Autodesk Inventor part; units mm, degrees
ref_plane "YZ Plane" through (0, 0, 0) normal (1, 0, 0) x (0, 1, 0)
ref_plane "XZ Plane" through (0, 0, 0) normal (0, 1, 0) x (-1, 0, 0)
ref_plane "XY Plane" through (0, 0, 0) normal (0, 0, 1) x (1, 0, 0)
sketch "Boceto1" plane through (0, 0, 0) normal (0, 0, 1) x (1, 0, 0)
  point P0 (0, 0)
sketch "Boceto2" plane through (0, 0, 0) normal (0, 0, 1) x (1, 0, 0)
  line L0 (-7.0268, -6.2798) -> (7.0268, -6.2798)
  line L1 (7.0268, -6.2798) -> (7.0268, 6.2798)
  line L2 (7.0268, 6.2798) -> (-7.0268, 6.2798)
  line L3 (-7.0268, 6.2798) -> (-7.0268, -6.2798)
  line L4 (-7.0268, -6.2798) -> (7.0268, 6.2798) construction
  line L5 (7.0268, -6.2798) -> (-7.0268, 6.2798) construction
  line L6 (-9.5542, -8.5385) -> (-9.5542, 8.5385)
  line L7 (-9.5542, 8.5385) -> (38.1222, 8.5385)
  line L8 (38.1222, 8.5385) -> (38.1222, -8.5385)
  line L9 (38.1222, -8.5385) -> (-9.5542, -8.5385)
  point P0 (0, 0)
extrude "Extrusión1" add sketch "Boceto2" along normal blind 5.08
Model file for the job. Use its own axes, mm. A direction names the side the tool comes from. Give positions to 0.01 mm unless a question says otherwise; leave off trailing zeros. Order: outer loops, then holes, each group sorted by start corner. A loop starts at its lowest first (then second) coordinate and runs counter-clockwise, first axis right, second up. Notation, with made-up numbers: M 48.5,-38.5 L 106.5,-38.5 A14 ccw 106.5,-24.5 Z; hole C -32.75,-38.5 d3. An arc over 180 degrees is marked long. Write item = value, one per line.
Q1. Cut at A-A, the plane y = 3.25. List the corners of the cut face in (x, z).
Derived:
outline = M -9.55,0 L -7.03,0 L -7.03,5.08 L -9.55,5.08 Z; M 7.03,0 L 38.12,0 L 38.12,5.08 L 7.03,5.08 Z
Q2. Cut at C-C, the plane x = 6. List the corners of the cut face in (y, z).
Derived:
outline = M -8.54,0 L -6.28,0 L -6.28,5.08 L -8.54,5.08 Z; M 6.28,0 L 8.54,0 L 8.54,5.08 L 6.28,5.08 Z
Q3. Drill centre lines: line 1 (Y direction, x = -2, z = 2.1); line 2 (X direction, y = 1.75, z = 0.85). Where is each one in solid material? Low to high. Write a range as [from, to].
Derived:
line_1 = [-8.54, -6.28], [6.28, 8.54]
line_2 = [-9.55, -7.03], [7.03, 38.12]
Q4. Tool access for faces 1 (the flat face through (7.027, 0, 3)), 2 (the flat face through (-9.554, 0, 3)): list every direction of +Z, -Z, +X, -X, +Y, -Y with a clear straight run to the whole face (end or side of a thin tool).
Derived:
face_1 = +Z, -Z
face_2 = +Z, -Z, -X, +Y, -Y
Q5. Cut at B-B, the plane z = 2.6. List the corners of the cut face in (x, y).
Derived:
outline = M -9.55,-8.54 L 38.12,-8.54 L 38.12,8.54 L -9.55,8.54 Z; hole M -7.03,-6.28 L 7.03,-6.28 L 7.03,6.28 L -7.03,6.28 Z
